Check sheet for the modelled part. Datum: model origin and axes. Units: mm. Face numbers are marked on the shaded views. Coordinates: 2 decimals unless noted, no trailing zeros. Loops run counter-clockwise (first coordinate to the right, second up) from the corner with the lowest first, then second, coordinate; pieces in that order, holes last. Notation, with made-up numbers: (69.25, 60) - (86.25, 60) arc R15 cw to (86.25, 82) - close; hole circle Ø1 at (54.25, 72.5). An arc over 180 degrees is marked (long way). Use a Markdown table: item, result. Add a question column.
1) Sectioned sample at A-A, the plane x = -30. Enter the section's corners in (y, z).
2) Thickness scan on line 1 (X direction, y = -0.9, z = -55); line 2 (X direction, y = 0.3, z = -41); line 3 (Z direction, x = 17, y = 3.4). Record the ranges inside material, lowest first.
3) Sectioned sample at B-B, the plane z = -55. Enter the section's corners in (x, y).
4) Go/stop test with flat-tipped pins: P1, Ø1, axis at x = -2.5, y = 1, coming from the -Z side; P2, Ø7.5, axis at x = -17.78, z = -30, coming from the +Y side; P3, Ø10, axis at x = 2.65, z = -9, coming from the -Y side; P4, Ø2, axis at y = 1, z = -34.5, coming from the +X side. Record where each tip stops, or that it passes through.
5) Draft check along Z on the marked faces 1 and 2. Enter one of: pulls with the +Z half, pulls with the -Z half, needs draft (parallel to the pull), parting line crosses it, or undercut.
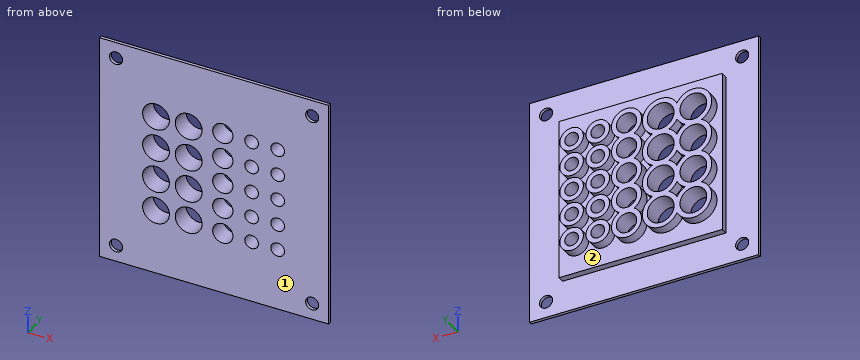
from build123d import *

# Parameters (mm, degrees)
SKETCH1_W           = 50
SKETCH1_H           = 50
SKETCH1_R           = 4.1
SKETCH1_R_2         = 3.1
SKETCH1_R_3         = 2.1
BOSS_EXTRUDE1_DEPTH = 1.5
SKETCH2_R           = 5.6
SKETCH2_R_2         = 4.1
SKETCH2_R_3         = 4.6
SKETCH2_R_4         = 3.1
SKETCH2_R_5         = 3.6
SKETCH2_R_6         = 2.1
EXTRUDE_THIN1_DEPTH = 3
SKETCH3_W           = 70
SKETCH3_H           = 70
SKETCH3_R           = 2
SKETCH3_W_2         = 50
SKETCH3_H_2         = 50
BOSS_EXTRUDE2_DEPTH = 1


with BuildPart() as part:
    # Sketch1 → Boss-Extrude1 (new, symmetric)
    with BuildSketch(Plane(origin=(0, 0, 0), x_dir=(1, 0, 0), z_dir=(0, 1, 0))):
        with Locations((0, 25)):
            Rectangle(SKETCH1_W, SKETCH1_H)
        with Locations(Location((-17.77819266, 10, 0), (0, 0, 270))):
            Circle(SKETCH1_R, mode=Mode.SUBTRACT)
        with Locations(Location((-17.77819266, 20, 0), (0, 0, 270))):
            Circle(SKETCH1_R, mode=Mode.SUBTRACT)
        with Locations(Location((-17.77819266, 30, 0), (0, 0, 270))):
            Circle(SKETCH1_R, mode=Mode.SUBTRACT)
        with Locations(Location((-17.77819266, 40, 0), (0, 0, 270))):
            Circle(SKETCH1_R, mode=Mode.SUBTRACT)
        with Locations(Location((2.654804044, 9, 0), (0, 0, 270))):
            Circle(SKETCH1_R_2, mode=Mode.SUBTRACT)
        with Locations(Location((2.654804044, 17, 0), (0, 0, 270))):
            Circle(SKETCH1_R_2, mode=Mode.SUBTRACT)
        with Locations(Location((2.654804044, 25, 0), (0, 0, 270))):
            Circle(SKETCH1_R_2, mode=Mode.SUBTRACT)
        with Locations(Location((2.654804044, 33, 0), (0, 0, 270))):
            Circle(SKETCH1_R_2, mode=Mode.SUBTRACT)
        with Locations(Location((2.654804044, 41, 0), (0, 0, 270))):
            Circle(SKETCH1_R_2, mode=Mode.SUBTRACT)
        with Locations(Location((11.466739275, 9, 0), (0, 0, 270))):
            Circle(SKETCH1_R_3, mode=Mode.SUBTRACT)
        with Locations(Location((19.466739275, 9, 0), (0, 0, 270))):
            Circle(SKETCH1_R_3, mode=Mode.SUBTRACT)
        with Locations(Location((19.466739275, 17, 0), (0, 0, 270))):
            Circle(SKETCH1_R_3, mode=Mode.SUBTRACT)
        with Locations(Location((19.466739275, 25, 0), (0, 0, 270))):
            Circle(SKETCH1_R_3, mode=Mode.SUBTRACT)
        with Locations(Location((19.466739275, 33, 0), (0, 0, 270))):
            Circle(SKETCH1_R_3, mode=Mode.SUBTRACT)
        with Locations(Location((19.466739275, 41, 0), (0, 0, 270))):
            Circle(SKETCH1_R_3, mode=Mode.SUBTRACT)
        with Locations(Location((11.466739275, 17, 0), (0, 0, 270))):
            Circle(SKETCH1_R_3, mode=Mode.SUBTRACT)
        with Locations(Location((11.466739275, 25, 0), (0, 0, 270))):
            Circle(SKETCH1_R_3, mode=Mode.SUBTRACT)
        with Locations(Location((11.466739275, 33, 0), (0, 0, 270))):
            Circle(SKETCH1_R_3, mode=Mode.SUBTRACT)
        with Locations(Location((11.466739275, 41, 0), (0, 0, 270))):
            Circle(SKETCH1_R_3, mode=Mode.SUBTRACT)
        with Locations(Location((-7.77819266, 10, 0), (0, 0, 270))):
            Circle(SKETCH1_R, mode=Mode.SUBTRACT)
        with Locations(Location((-7.77819266, 20, 0), (0, 0, 270))):
            Circle(SKETCH1_R, mode=Mode.SUBTRACT)
        with Locations(Location((-7.77819266, 30, 0), (0, 0, 270))):
            Circle(SKETCH1_R, mode=Mode.SUBTRACT)
        with Locations(Location((-7.77819266, 40, 0), (0, 0, 270))):
            Circle(SKETCH1_R, mode=Mode.SUBTRACT)
    extrude(amount=BOSS_EXTRUDE1_DEPTH, both=True)

    # Sketch2 → Extrude-Thin1 (add)
    # profile 1 of 23: a face of its own
    with BuildSketch(Plane(origin=(0, 1.5, 0), x_dir=(1, 0, 0), z_dir=(0, 1, 0))):
        with Locations((-17.77819266, 10)):
            Circle(SKETCH2_R)
        with Locations((-17.77819266, 10)):
            Circle(SKETCH2_R_2, mode=Mode.SUBTRACT)
    # profile 2 of 23: a face of its own
    with BuildSketch(Plane(origin=(0, 1.5, 0), x_dir=(1, 0, 0), z_dir=(0, 1, 0))):
        with Locations((-17.77819266, 20)):
            Circle(SKETCH2_R)
        with Locations((-17.77819266, 20)):
            Circle(SKETCH2_R_2, mode=Mode.SUBTRACT)
    # profile 3 of 23: a face of its own
    with BuildSketch(Plane(origin=(0, 1.5, 0), x_dir=(1, 0, 0), z_dir=(0, 1, 0))):
        with Locations((-17.77819266, 30)):
            Circle(SKETCH2_R)
        with Locations((-17.77819266, 30)):
            Circle(SKETCH2_R_2, mode=Mode.SUBTRACT)
    # profile 4 of 23: a face of its own
    with BuildSketch(Plane(origin=(0, 1.5, 0), x_dir=(1, 0, 0), z_dir=(0, 1, 0))):
        with Locations((2.654804044, 17)):
            Circle(SKETCH2_R_3)
        with Locations((2.654804044, 17)):
            Circle(SKETCH2_R_4, mode=Mode.SUBTRACT)
    # profile 5 of 23: a face of its own
    with BuildSketch(Plane(origin=(0, 1.5, 0), x_dir=(1, 0, 0), z_dir=(0, 1, 0))):
        with Locations((-17.77819266, 40)):
            Circle(SKETCH2_R)
        with Locations((-17.77819266, 40)):
            Circle(SKETCH2_R_2, mode=Mode.SUBTRACT)
    # profile 6 of 23: a face of its own
    with BuildSketch(Plane(origin=(0, 1.5, 0), x_dir=(1, 0, 0), z_dir=(0, 1, 0))):
        with Locations((2.654804044, 9)):
            Circle(SKETCH2_R_3)
        with Locations((2.654804044, 9)):
            Circle(SKETCH2_R_4, mode=Mode.SUBTRACT)
    # profile 7 of 23: a face of its own
    with BuildSketch(Plane(origin=(0, 1.5, 0), x_dir=(1, 0, 0), z_dir=(0, 1, 0))):
        with Locations((2.654804044, 25)):
            Circle(SKETCH2_R_3)
        with Locations((2.654804044, 25)):
            Circle(SKETCH2_R_4, mode=Mode.SUBTRACT)
    # profile 8 of 23: a face of its own
    with BuildSketch(Plane(origin=(0, 1.5, 0), x_dir=(1, 0, 0), z_dir=(0, 1, 0))):
        with Locations((2.654804044, 33)):
            Circle(SKETCH2_R_3)
        with Locations((2.654804044, 33)):
            Circle(SKETCH2_R_4, mode=Mode.SUBTRACT)
    # profile 9 of 23: a face of its own
    with BuildSketch(Plane(origin=(0, 1.5, 0), x_dir=(1, 0, 0), z_dir=(0, 1, 0))):
        with Locations((2.654804044, 41)):
            Circle(SKETCH2_R_3)
        with Locations((2.654804044, 41)):
            Circle(SKETCH2_R_4, mode=Mode.SUBTRACT)
    # profile 10 of 23: a face of its own
    with BuildSketch(Plane(origin=(0, 1.5, 0), x_dir=(1, 0, 0), z_dir=(0, 1, 0))):
        with Locations((11.466739275, 9)):
            Circle(SKETCH2_R_5)
        with Locations((11.466739275, 9)):
            Circle(SKETCH2_R_6, mode=Mode.SUBTRACT)
    # profile 11 of 23: a face of its own
    with BuildSketch(Plane(origin=(0, 1.5, 0), x_dir=(1, 0, 0), z_dir=(0, 1, 0))):
        with Locations((-7.77819266, 10)):
            Circle(SKETCH2_R)
        with Locations((-7.77819266, 10)):
            Circle(SKETCH2_R_2, mode=Mode.SUBTRACT)
    # profile 12 of 23: a face of its own
    with BuildSketch(Plane(origin=(0, 1.5, 0), x_dir=(1, 0, 0), z_dir=(0, 1, 0))):
        with Locations((19.466739275, 9)):
            Circle(SKETCH2_R_5)
        with Locations((19.466739275, 9)):
            Circle(SKETCH2_R_6, mode=Mode.SUBTRACT)
    # profile 13 of 23: a face of its own
    with BuildSketch(Plane(origin=(0, 1.5, 0), x_dir=(1, 0, 0), z_dir=(0, 1, 0))):
        with Locations((19.466739275, 17)):
            Circle(SKETCH2_R_5)
        with Locations((19.466739275, 17)):
            Circle(SKETCH2_R_6, mode=Mode.SUBTRACT)
    # profile 14 of 23: a face of its own
    with BuildSketch(Plane(origin=(0, 1.5, 0), x_dir=(1, 0, 0), z_dir=(0, 1, 0))):
        with Locations((19.466739275, 25)):
            Circle(SKETCH2_R_5)
        with Locations((19.466739275, 25)):
            Circle(SKETCH2_R_6, mode=Mode.SUBTRACT)
    # profile 15 of 23: a face of its own
    with BuildSketch(Plane(origin=(0, 1.5, 0), x_dir=(1, 0, 0), z_dir=(0, 1, 0))):
        with Locations((19.466739275, 33)):
            Circle(SKETCH2_R_5)
        with Locations((19.466739275, 33)):
            Circle(SKETCH2_R_6, mode=Mode.SUBTRACT)
    # profile 16 of 23: a face of its own
    with BuildSketch(Plane(origin=(0, 1.5, 0), x_dir=(1, 0, 0), z_dir=(0, 1, 0))):
        with Locations((19.466739275, 41)):
            Circle(SKETCH2_R_5)
        with Locations((19.466739275, 41)):
            Circle(SKETCH2_R_6, mode=Mode.SUBTRACT)
    # profile 17 of 23: a face of its own
    with BuildSketch(Plane(origin=(0, 1.5, 0), x_dir=(1, 0, 0), z_dir=(0, 1, 0))):
        with Locations((11.466739275, 17)):
            Circle(SKETCH2_R_5)
        with Locations((11.466739275, 17)):
            Circle(SKETCH2_R_6, mode=Mode.SUBTRACT)
    # profile 18 of 23: a face of its own
    with BuildSketch(Plane(origin=(0, 1.5, 0), x_dir=(1, 0, 0), z_dir=(0, 1, 0))):
        with Locations((11.466739275, 25)):
            Circle(SKETCH2_R_5)
        with Locations((11.466739275, 25)):
            Circle(SKETCH2_R_6, mode=Mode.SUBTRACT)
    # profile 19 of 23: a face of its own
    with BuildSketch(Plane(origin=(0, 1.5, 0), x_dir=(1, 0, 0), z_dir=(0, 1, 0))):
        with Locations((11.466739275, 33)):
            Circle(SKETCH2_R_5)
        with Locations((11.466739275, 33)):
            Circle(SKETCH2_R_6, mode=Mode.SUBTRACT)
    # profile 20 of 23: a face of its own
    with BuildSketch(Plane(origin=(0, 1.5, 0), x_dir=(1, 0, 0), z_dir=(0, 1, 0))):
        with Locations((11.466739275, 41)):
            Circle(SKETCH2_R_5)
        with Locations((11.466739275, 41)):
            Circle(SKETCH2_R_6, mode=Mode.SUBTRACT)
    # profile 21 of 23: a face of its own
    with BuildSketch(Plane(origin=(0, 1.5, 0), x_dir=(1, 0, 0), z_dir=(0, 1, 0))):
        with Locations((-7.77819266, 20)):
            Circle(SKETCH2_R)
        with Locations((-7.77819266, 20)):
            Circle(SKETCH2_R_2, mode=Mode.SUBTRACT)
    # profile 22 of 23: a face of its own
    with BuildSketch(Plane(origin=(0, 1.5, 0), x_dir=(1, 0, 0), z_dir=(0, 1, 0))):
        with Locations((-7.77819266, 30)):
            Circle(SKETCH2_R)
        with Locations((-7.77819266, 30)):
            Circle(SKETCH2_R_2, mode=Mode.SUBTRACT)
    # profile 23 of 23: a face of its own
    with BuildSketch(Plane(origin=(0, 1.5, 0), x_dir=(1, 0, 0), z_dir=(0, 1, 0))):
        with Locations((-7.77819266, 40)):
            Circle(SKETCH2_R)
        with Locations((-7.77819266, 40)):
            Circle(SKETCH2_R_2, mode=Mode.SUBTRACT)
    extrude(amount=EXTRUDE_THIN1_DEPTH)

    # Sketch3 → Boss-Extrude2 (add)
    with BuildSketch(Plane.XZ.offset(1.5)):
        with Locations((0, -25)):
            Rectangle(SKETCH3_W, SKETCH3_H)
        with Locations(Location((-30, 5, 0), (0, 0, 270))):
            Circle(SKETCH3_R, mode=Mode.SUBTRACT)
        with Locations(Location((30, 5, 0), (0, 0, 270))):
            Circle(SKETCH3_R, mode=Mode.SUBTRACT)
        with Locations(Location((30, -55, 0), (0, 0, 270))):
            Circle(SKETCH3_R, mode=Mode.SUBTRACT)
        with Locations(Location((-30, -55, 0), (0, 0, 270))):
            Circle(SKETCH3_R, mode=Mode.SUBTRACT)
        with Locations((0, -25)):
            Rectangle(SKETCH3_W_2, SKETCH3_H_2, mode=Mode.SUBTRACT)
    extrude(amount=-BOSS_EXTRUDE2_DEPTH)


solid = part.part
Solved:
| question | item | result |
|---|---|---|
| 1 | outline | (-1.5, -60) - (-0.5, -60) - (-0.5, -57) - (-1.5, -57) - close; (-1.5, -53) - (-0.5, -53) - (-0.5, 3) - (-1.5, 3) - close; (-1.5, 7) - (-0.5, 7) - (-0.5, 10) - (-1.5, 10) - close |
| 2 | line 1 | x = -35 to -32, -28 to 28, 32 to 35 |
| 2 | line 2 | x = -25 to -21.75, -13.8 to -11.75, -3.8 to -0.45, 5.75 to 9.37, 13.57 to 17.37, 21.57 to 25 |
| 2 | line 3 | z = -43.62 to -38.38, -35.62 to -30.38, -27.62 to -22.38, -19.62 to -14.38, -11.62 to -6.38 |
| 3 | outline | (-35, -1.5) - (-32, -1.5) - (-32, -0.5) - (-35, -0.5) - close; (-28, -1.5) - (28, -1.5) - (28, -0.5) - (-28, -0.5) - close; (32, -1.5) - (35, -1.5) - (35, -0.5) - (32, -0.5) - close |
| 4 | P1 | stops at z = -50 |
| 4 | P2 | passes through |
| 4 | P3 | stops at y = -1.5 |
| 4 | P4 | stops at x = 25 |
| 5 | face 1 | needs draft |
| 5 | face 2 | undercut |
